The model under review builds one solid part; all positions refer to its coordinate system, in mm. Face numbers are marked on the shaded views. A direction names the side the tool comes from. Give positions to 0.01 mm unless a question says otherwise; leave off trailing zeros. Order: outer loops, then holes, each group sorted by start corner. A loop starts at its lowest first (then second) coordinate and runs counter-clockwise, first axis right, second up. Notation, with made-up numbers: M 61,19.5 L 113,19.5 A26 ccw 113,55.5 Z; hole C 79,36.5 d10. An arc over 180 degrees is marked long. One line per question, with ' | ' between items. Start each with the question number.
1. We need section B-B on x = 14. Write out the cut boundary in (y, z), then the cut area to 3 significant figures.
2. We need section D-D on y = -5. Write out the cut boundary in (x, z), then the cut area to 3 significant figures.
3. For the marked faces 1 and 2, list the 3-axis set-ups (+Z, -Z, +X, -X, +Y, -Y) from which the entire face can be reached by the end or side of a thin tool; tool diameter is ignored.
4. We need section A-A on y = -17.5. Write out the cut boundary in (x, z).
5. Insertion check: P1, Ø12, axis at x = 2, z = 4, coming from the -Y side; P2, Ø6.5, axis at x = -4, y = 4.5, coming from the -Z side; P3, Ø6.5, axis at x = 0, y = -17.5, coming from the +Z side. Each pin has a flat end and moves straight along its axis. Give the tip position at first contact, or say it passes through.
6. We need section C-C on z = 39. Count the separate pieces of the cut face and the enclosed holes in it, then the cut area to 3 significant figures.
7. Wall thickness on L1, parallel to Y at x = 0, z = 26.9; L2, parallel to Z at x = 1, y = 13; L3, parallel to Z at x = -1.5, y = 10: over which ranges is each line inside the solid? List them lowest first.
```python
from build123d import *

# Parameters (mm, degrees)
IZIM1_R                     = 11
Y_KSEKLIK_EKSTR_ZYON1_DEPTH = 28
IZIM2_R                     = 22
Y_KSEKLIK_EKSTR_ZYON2_DEPTH = 2.4
IZIM3_R                     = 2.5
KES_EKSTR_ZYON1_DEPTH       = 10
IZIM4_R                     = 3.9
Y_KSEKLIK_EKSTR_ZYON3_DEPTH = 9
IZIM6_R                     = 3.25
KES_EKSTR_ZYON3_DEPTH       = 2
IZIM7_R                     = 0.5
Y_KSEKLIK_EKSTR_ZYON5_DEPTH = 6
IZIM8_R                     = 0.35
Y_KSEKLIK_EKSTR_ZYON6_DEPTH = 4
IZIM9_R                     = 2
KES_EKSTR_ZYON4_DEPTH       = 2
IZIM10_R                    = 0.5
Y_KSEKLIK_EKSTR_ZYON7_DEPTH = 6
IZIM12_R                    = 9
IZIM12_R_2                  = 7.5
KES_EKSTR_ZYON5_DEPTH       = 4
IZIM13_R                    = 0.35
Y_KSEKLIK_EKSTR_ZYON8_DEPTH = 4


with BuildPart() as part:
    # Çizim1 → Yükseklik-Ekstrüzyon1 (new body)
    with BuildSketch(Plane.XY):
        Circle(IZIM1_R)
    extrude(amount=Y_KSEKLIK_EKSTR_ZYON1_DEPTH)

    # Çizim2 → Yükseklik-Ekstrüzyon2 (add)
    with BuildSketch(Plane.XY.offset(23)):
        Circle(IZIM2_R)
    extrude(amount=-Y_KSEKLIK_EKSTR_ZYON2_DEPTH)

    # Çizim3 → Kes-Ekstrüzyon1 (cut)
    with BuildSketch(Plane.XY.offset(23)):
        with Locations((0, -17.5)):
            Circle(IZIM3_R)
        with Locations((-15.155444566, 8.75)):
            Circle(IZIM3_R)
        with Locations((15.155444566, 8.75)):
            Circle(IZIM3_R)
    extrude(amount=-KES_EKSTR_ZYON1_DEPTH, mode=Mode.SUBTRACT)

    # Çizim4 → Yükseklik-Ekstrüzyon3 (add)
    with BuildSketch(Plane.XY.offset(28)):
        Circle(IZIM4_R)
    extrude(amount=Y_KSEKLIK_EKSTR_ZYON3_DEPTH)

    # Çizim6 → Kes-Ekstrüzyon3 (cut)
    with BuildSketch(Plane.XY.offset(37)):
        Circle(IZIM6_R)
    extrude(amount=-KES_EKSTR_ZYON3_DEPTH, mode=Mode.SUBTRACT)

    # Çizim7 → Yükseklik-Ekstrüzyon5 (add)
    with BuildSketch(Plane.XY.offset(35)):
        with Locations((0, 2.5)):
            Circle(IZIM7_R)
        with Locations((1.25, 2.165063509)):
            Circle(IZIM7_R)
        with Locations((2.165063509, 1.25)):
            Circle(IZIM7_R)
        with Locations((2.5, 0)):
            Circle(IZIM7_R)
        with Locations((2.165063509, -1.25)):
            Circle(IZIM7_R)
        with Locations((1.25, -2.165063509)):
            Circle(IZIM7_R)
        with Locations((0, -2.5)):
            Circle(IZIM7_R)
        with Locations((-1.25, -2.165063509)):
            Circle(IZIM7_R)
        with Locations((-2.165063509, -1.25)):
            Circle(IZIM7_R)
        with Locations((-2.5, 0)):
            Circle(IZIM7_R)
        with Locations((-2.165063509, 1.25)):
            Circle(IZIM7_R)
        with Locations((-1.25, 2.165063509)):
            Circle(IZIM7_R)
    extrude(amount=Y_KSEKLIK_EKSTR_ZYON5_DEPTH)

    # Çizim8 → Yükseklik-Ekstrüzyon6 (add)
    with BuildSketch(Plane.XY.offset(41)):
        with Locations((0, 2.5)):
            Circle(IZIM8_R)
        with Locations((1.25, 2.165063509)):
            Circle(IZIM8_R)
        with Locations((2.165063509, 1.25)):
            Circle(IZIM8_R)
        with Locations((2.5, 0)):
            Circle(IZIM8_R)
        with Locations((2.165063509, -1.25)):
            Circle(IZIM8_R)
        with Locations((1.25, -2.165063509)):
            Circle(IZIM8_R)
        with Locations((0, -2.5)):
            Circle(IZIM8_R)
        with Locations((-1.25, -2.165063509)):
            Circle(IZIM8_R)
        with Locations((-2.165063509, -1.25)):
            Circle(IZIM8_R)
        with Locations((-2.5, 0)):
            Circle(IZIM8_R)
        with Locations((-2.165063509, 1.25)):
            Circle(IZIM8_R)
        with Locations((-1.25, 2.165063509)):
            Circle(IZIM8_R)
    extrude(amount=Y_KSEKLIK_EKSTR_ZYON6_DEPTH)

    # Çizim9 → Kes-Ekstrüzyon4 (cut)
    with BuildSketch(Plane(origin=(0, 0, 0), x_dir=(-1, 0, 0), z_dir=(0, 0, -1))):
        with Locations((-7.5, 0)):
            Circle(IZIM9_R)
        with Locations((7.5, 0)):
            Circle(IZIM9_R)
    extrude(amount=-KES_EKSTR_ZYON4_DEPTH, mode=Mode.SUBTRACT)

    # Çizim10 → Yükseklik-Ekstrüzyon7 (add)
    with BuildSketch(Plane(origin=(0, 0, 2), x_dir=(-1, 0, 0), z_dir=(0, 0, -1))):
        with Locations((7.5, 1.25)):
            Circle(IZIM10_R)
        with Locations((8.582531755, 0.625)):
            Circle(IZIM10_R)
        with Locations((8.582531755, -0.625)):
            Circle(IZIM10_R)
        with Locations((7.5, -1.25)):
            Circle(IZIM10_R)
        with Locations(Location((-6.417468245, 0.625, 0), (0, 0, 180))):
            Circle(IZIM10_R)
        with Locations(Location((-6.417468245, -0.625, 0), (0, 0, 180))):
            Circle(IZIM10_R)
        with Locations(Location((-7.5, -1.25, 0), (0, 0, 180))):
            Circle(IZIM10_R)
        with Locations(Location((-8.582531755, -0.625, 0), (0, 0, 180))):
            Circle(IZIM10_R)
        with Locations((6.417468245, -0.625)):
            Circle(IZIM10_R)
        with Locations((6.417468245, 0.625)):
            Circle(IZIM10_R)
        with Locations(Location((-8.582531755, 0.625, 0), (0, 0, 180))):
            Circle(IZIM10_R)
        with Locations(Location((-7.5, 1.25, 0), (0, 0, 180))):
            Circle(IZIM10_R)
    extrude(amount=Y_KSEKLIK_EKSTR_ZYON7_DEPTH)

    # Çizim12 → Kes-Ekstrüzyon5 (cut)
    with BuildSketch(Plane.XY.offset(28)):
        Circle(IZIM12_R)
        Circle(IZIM12_R_2, mode=Mode.SUBTRACT)
    extrude(amount=-KES_EKSTR_ZYON5_DEPTH, mode=Mode.SUBTRACT)

    # Çizim13 → Yükseklik-Ekstrüzyon8 (add)
    with BuildSketch(Plane(origin=(0, 0, -4), x_dir=(-1, 0, 0), z_dir=(0, 0, -1))):
        with Locations((7.5, 1.25)):
            Circle(IZIM13_R)
        with Locations((8.582531755, 0.625)):
            Circle(IZIM13_R)
        with Locations((8.582531755, -0.625)):
            Circle(IZIM13_R)
        with Locations((7.5, -1.25)):
            Circle(IZIM13_R)
        with Locations((6.417468245, -0.625)):
            Circle(IZIM13_R)
        with Locations((6.417468245, 0.625)):
            Circle(IZIM13_R)
        with Locations(Location((-6.417468245, 0.625, 0), (0, 0, 180))):
            Circle(IZIM13_R)
        with Locations(Location((-6.417468245, -0.625, 0), (0, 0, 180))):
            Circle(IZIM13_R)
        with Locations(Location((-7.5, -1.25, 0), (0, 0, 180))):
            Circle(IZIM13_R)
        with Locations(Location((-8.582531755, -0.625, 0), (0, 0, 180))):
            Circle(IZIM13_R)
        with Locations(Location((-8.582531755, 0.625, 0), (0, 0, 180))):
            Circle(IZIM13_R)
        with Locations(Location((-7.5, 1.25, 0), (0, 0, 180))):
            Circle(IZIM13_R)
    extrude(amount=Y_KSEKLIK_EKSTR_ZYON8_DEPTH)


solid = part.part
```
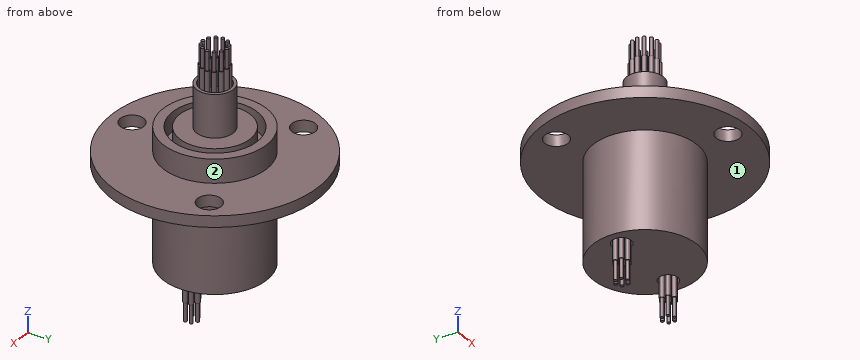
Entries:
1) outline: M -16.97,20.6 L 6.53,20.6 L 6.53,23 L -16.97,23 Z; M 10.97,20.6 L 16.97,20.6 L 16.97,23 L 10.97,23 Z | area: 70.8 mm^2
2) outline: M -21.42,20.6 L -9.8,20.6 L -9.8,0 L 9.8,0 L 9.8,20.6 L 21.42,20.6 L 21.42,23 L 9.8,23 L 9.8,28 L 7.48,28 L 7.48,24 L 5.59,24 L 5.59,28 L -5.59,28 L -5.59,24 L -7.48,24 L -7.48,28 L -9.8,28 L -9.8,23 L -21.42,23 Z | area: 589 mm^2
3) face 1: -Z | face 2: +Z
4) outline: M -13.33,20.6 L -2.5,20.6 L -2.5,23 L -13.33,23 Z; M 2.5,20.6 L 13.33,20.6 L 13.33,23 L 2.5,23 Z
5) P1: stops at y = -11 | P2: stops at z = 0 | P3: stops at z = 23
6) separate pieces: 12 | enclosed holes: 0 | area: 9.42 mm^2
7) L1: y = -11 to -9, -7.5 to 7.5, 9 to 11 | L2: z = 20.6 to 23 | L3: z = 0 to 28
